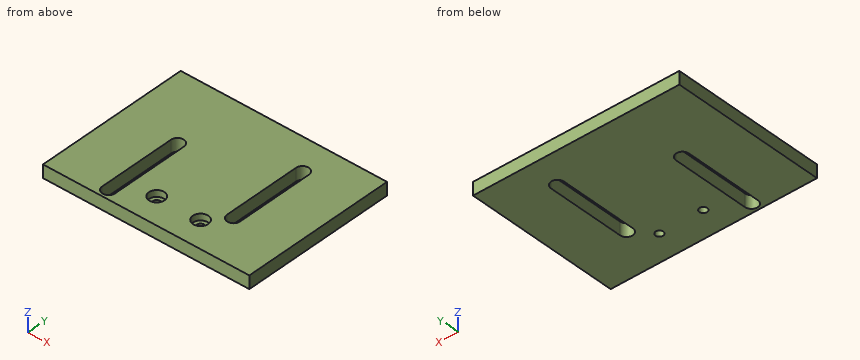
Autodesk Inventor part; units mm, degrees
ref_plane "YZ Plane" through (0, 0, 0) normal (1, 0, 0) x (0, 1, 0)
ref_plane "XZ Plane" through (0, 0, 0) normal (0, 1, 0) x (-1, 0, 0)
ref_plane "XY Plane" through (0, 0, 0) normal (0, 0, 1) x (1, 0, 0)
sketch "Sketch1" plane through (0, 0, 0) normal (0, 0, 1) x (1, 0, 0)
  line L0 (-401.966, 248.4646) -> (398.034, 248.4646)
  line L1 (398.034, 248.4646) -> (398.034, -251.5354)
  line L2 (398.034, -251.5354) -> (-401.966, -251.5354)
  line L3 (-401.966, -251.5354) -> (-401.966, 248.4646)
  dimension "d0" = 800
  dimension "d1" = 500
  dimension "d2" = 800
extrude "Extrusion1" add sketch "Sketch1" along normal blind 5
sketch "Sketch2" plane through (0, 0, 5) normal (0, 0, 1) x (1, 0, 0)
  point P0 (0, 0)
sketch "Sketch3" plane through (0, 0, 5) normal (0, 0, 1) x (1, 0, 0)
  line L0 (-401.966, -251.5354) -> (398.034, -251.5354)
  point P0 (0, 0)
sketch "Sketch4" plane through (0, 0, 5) normal (0, 0, 1) x (1, 0, 0)
  line L0 (-401.966, -251.5354) -> (398.034, -251.5354)
  line L1 (-1.966, -251.5354) -> (-1.966, -241.0354)
  line L2 (-1.966, -241.0354) -> (6.534, -241.0354)
  line L3 (-1.966, -241.0354) -> (-10.466, -241.0354)
  point P0 (0, 0)
  dimension "d7" = 10.5
  dimension "d8" = 8.5
  dimension "d9" = 8.5
hole "Hole1" at (6.534, -241.0354, 5) at (-10.466, -241.0354, 5) direction (0, 0, -1) diameter 3 depth 5 tip angle 118 counterbore diameter 6 counterbore depth 2.5
sketch "Sketch5" plane through (0, 0, 5) normal (0, 0, 1) x (1, 0, 0)
  point P0 (0, 0)
sketch "Sketch6" plane through (0, 0, 5) normal (0, 0, 1) x (1, 0, 0)
  line L0 (398.034, -251.5354) -> (-401.966, -251.5354)
  line L1 (6.5526, -251.5354) -> (6.5526, -248.0354)
  line L2 (0, -251.5354) -> (3.5, -251.5354) construction
  line L3 (-4.8949, -248.0354) -> (13.1051, -248.0354)
  line L4 (-4.8949, -248.0354) -> (-22.8949, -248.0354)
  line L5 (13.1051, -248.0354) -> (13.1051, -234.0354)
  circle A0 centre (-10.466, -241.0354) radius 1.5
  line L6 (-10.466, -241.0354) -> (-16.966, -241.0354)
  line L7 (6.5526, -241.0354) -> (13.0526, -241.0354)
  line L8 (-22.8949, -248.0354) -> (-20.3949, -248.0354)
  line L9 (-20.3949, -248.0354) -> (-20.3949, -218.0354)
  line L10 (-20.3949, -218.0354) -> (-22.8949, -218.0354)
  line L11 (-22.8949, -218.0354) -> (-22.8949, -248.0354)
  line L12 (-22.8949, -248.0354) -> (-25.3949, -248.0354)
  line L13 (-25.3949, -248.0354) -> (-25.3949, -218.0354)
  line L14 (-25.3949, -218.0354) -> (-22.8949, -218.0354)
  line L15 (-22.8949, -218.0354) -> (-22.8949, -248.0354)
  line L16 (13.1051, -234.0354) -> (15.6051, -234.0354)
  line L17 (15.6051, -234.0354) -> (15.6051, -204.0354)
  line L18 (15.6051, -204.0354) -> (13.1051, -204.0354)
  line L19 (13.1051, -204.0354) -> (13.1051, -234.0354)
  line L20 (13.1051, -234.0354) -> (10.6051, -234.0354)
  line L21 (10.6051, -234.0354) -> (10.6051, -204.0354)
  line L22 (10.6051, -204.0354) -> (13.1051, -204.0354)
  line L23 (13.1051, -204.0354) -> (13.1051, -234.0354)
  point P0 (0, 0)
  dimension "d17" = 3.5
  dimension "d18" = 90
  dimension "d19" = 18
  dimension "d20" = 18
  dimension "d21" = 14
  dimension "d22" = 6.5
  dimension "d23" = 6.5
  dimension "d24" = 2.5
  dimension "d25" = 30
  dimension "d26" = 2.5
  dimension "d27" = 2.5
  dimension "d28" = 30
  dimension "d29" = 2.5
  dimension "d30" = 30
  dimension "d52" = 36
  dimension "d53" = 17.0186
sketch "Sketch7" plane through (0, 0, 0) normal (0, 0, -1) x (-1, 0, 0)
  point P0 (0, 0)
hole "Hole2" at (-22.8949, -248.0354, 5) at (13.1051, -234.0354, 5) direction (0, 0, -1) diameter 5 depth 15 tip angle 118
extrude "Extrusion2" cut sketch "Sketch6" against normal blind 15 contours L20 L21 L22 L19 | L19 L18 L17 L16 | L4 L11 L10 L9 | L12 L13 L14 L11
hole "Hole3" at (-22.8949, -218.0354, 5) at (13.1051, -204.0354, 5) direction (0, 0, -1) diameter 5 depth 15 tip angle 118
sketch "Sketch8" plane through (0, 0, 5) normal (0, 0, 1) x (1, 0, 0)
  line L0 (398.034, -251.5354) -> (-401.966, -251.5354)
  line L1 (-45.2231, -251.5354) -> (34.7769, -251.5354)
  line L2 (34.7769, -251.5354) -> (34.7769, -191.5354)
  line L3 (34.7769, -191.5354) -> (-45.2231, -191.5354)
  line L4 (-45.2231, -191.5354) -> (-45.2231, -251.5354)
  line L5 (-45.2231, 276.0506) -> (-471.5877, 276.0506)
  line L6 (-471.5877, 276.0506) -> (-471.5877, -297.567)
  line L7 (-471.5877, -297.567) -> (-45.2231, -297.567)
  line L8 (-45.2231, -297.567) -> (-45.2231, 276.0506)
  line L9 (-45.2231, -191.5354) -> (471.8148, -191.5354)
  line L10 (471.8148, -191.5354) -> (471.8148, 308.5195)
  line L11 (471.8148, 308.5195) -> (-45.2231, 308.5195)
  line L12 (-45.2231, 308.5195) -> (-45.2231, -191.5354)
  line L13 (34.7769, -191.5354) -> (471.8148, -191.5354)
  line L14 (471.8148, -191.5354) -> (471.8148, -324.6244)
  line L15 (471.8148, -324.6244) -> (34.7769, -324.6244)
  line L16 (34.7769, -324.6244) -> (34.7769, -191.5354)
  point P0 (0, 0)
  dimension "d48" = 80
  dimension "d49" = 60
extrude "Extrusion3" cut sketch "Sketch8" against normal blind 15 contours L2 L9 L14 L15 L16 | L8 L7 L6 L5 L4 | L3 L8 L12 L11 L10 L9
properties part number "regla_digital"
Geometry check sheet. Reference: the model listing, model coordinates, mm. Round coordinates to 2 decimals unless told otherwise and drop trailing zeros. Loops run counter-clockwise (first coordinate to the right, second up) from the corner with the lowest first, then second, coordinate; pieces in that order, holes last. Notation, with made-up numbers: (-5.5, 68) -> (34.5, 68) arc R13 cw to (34.5, 80) -> close; hole circle Ø5 at (-10.75, 39). An arc over 180 degrees is marked (long way). Answer as a JSON object with one key per item and string values. Group by question number.
Item 1: Cross-section at B-B, the plane y = -230. Record the cut outline in (x, z).
Item 2: Cross-section at C-C, the plane z = 3.45. Record the cut outline in (x, y), plus the area to 3 significant figures.
Item 3: Cross-section at A-A, the plane y = -205.5. Record the cut outline in (x, z).
Item 4: Cross-section at D-D, the plane x = 14. Record the cut outline in (y, z), plus the area to 3 significant figures.
Item 5: Thickness scan on line 1 along X through (y, z) = (-221, 2.3); line 2 along X through (y, z) = (-243, 4.4); line 3 along X through (y, z) = (-243.5, 2.95). Record the ranges inside material, lowest first.
Item 6: Depth check by flat-ended pin: pin 1 Ø3 at (x, y) = (7, -242) entering from +Z. Enter the tip coordinate at first touch or a pass-through.
Determined:
{
 "1": {"outline": "(-45.22, 0) -> (-25.39, 0) -> (-25.39, 5) -> (-45.22, 5) -> close; (-20.39, 0) -> (10.61, 0) -> (10.61, 5) -> (-20.39, 5) -> close; (15.61, 0) -> (34.78, 0) -> (34.78, 5) -> (15.61, 5) -> close"},
 "2": {"outline": "(-45.22, -251.54) -> (34.78, -251.54) -> (34.78, -191.54) -> (-45.22, -191.54) -> close; hole (-25.39, -248.04) arc R2.5 ccw to (-20.39, -248.04) -> (-20.39, -218.04) arc R2.5 ccw to (-25.39, -218.04) -> close; hole circle Ø6 at (-10.47, -241.04); hole circle Ø6 at (6.53, -241.04); hole (10.61, -234.04) arc R2.5 ccw to (15.61, -234.04) -> (15.61, -204.04) arc R2.5 ccw to (10.61, -204.04) -> close", "area": "4,400 mm²"},
 "3": {"outline": "(-45.22, 0) -> (10.61, 0) -> (10.61, 5) -> (-45.22, 5) -> close; (15.61, 0) -> (34.78, 0) -> (34.78, 5) -> (15.61, 5) -> close"},
 "4": {"outline": "(-251.54, 0) -> (-236.37, 0) -> (-236.37, 5) -> (-251.54, 5) -> close; (-201.7, 0) -> (-191.54, 0) -> (-191.54, 5) -> (-201.7, 5) -> close", "area": "127 mm²"},
 "5": {"line 1": "x = -45.22 to -25.39, -20.39 to 10.61, 15.61 to 34.78", "line 2": "x = -45.22 to -25.39, -20.39 to -12.73, -8.2 to 4.27, 8.8 to 34.78", "line 3": "x = -45.22 to -25.39, -20.39 to -12.18, -8.76 to 4.82, 8.24 to 34.78"},
 "6": {"pin 1": "stops at z = 2.5"}
}
